Autodesk Inventor part; units mm, degrees
ref_plane "YZ Plane" through (0, 0, 0) normal (1, 0, 0) x (0, 1, 0)
ref_plane "XZ Plane" through (0, 0, 0) normal (0, 1, 0) x (-1, 0, 0)
ref_plane "XY Plane" through (0, 0, 0) normal (0, 0, 1) x (1, 0, 0)
sketch "Boceto1" plane through (0, 0, 0) normal (0, 0, 1) x (1, 0, 0)
  line L0 (0.9, -2.4) -> (-0.9, -2.4)
  line L1 (-0.9, -2.4) -> (-0.9, 2.4)
  line L2 (-0.9, 2.4) -> (0.9, 2.4)
  line L3 (0.9, 2.4) -> (0.9, -2.4)
  line L4 (0.9, -2.4) -> (-0.9, 2.4) construction
  line L5 (-0.9, -2.4) -> (0.9, 2.4) construction
  line L6 (2.4, -0.9) -> (-2.4, -0.9)
  line L7 (-2.4, -0.9) -> (-2.4, 0.9)
  line L8 (-2.4, 0.9) -> (2.4, 0.9)
  line L9 (2.4, 0.9) -> (2.4, -0.9)
  line L10 (2.4, -0.9) -> (-2.4, 0.9) construction
  line L11 (-2.4, -0.9) -> (2.4, 0.9) construction
  circle A0 centre (0, 0) radius 1.4
  point P0 (1.0724, 0.9)
  point P1 (0.9, 1.0724)
  point P2 (-0.9, 1.0724)
  point P3 (-1.0724, 0.9)
  point P4 (-1.0724, -0.9)
  point P5 (-0.9, -1.0724)
  point P6 (0.9, -1.0724)
  point P7 (1.0724, -0.9)
  dimension "d0" = 1.8
  dimension "d1" = 4.8
  dimension "d2" = 2.8
extrude "Extrusión1" add sketch "Boceto1" along normal blind 53
chamfer "Chaflán1" distance 0.2 angle 45 8 edges at (0.9, 2.4, 26.5) (2.4, 0.9, 26.5) (2.4, -0.9, 26.5) (0.9, -2.4, 26.5) (-0.9, 2.4, 26.5) (-2.4, 0.9, 26.5) (-2.4, -0.9, 26.5) (-0.9, -2.4, 26.5)
properties part number "EjeMotor"
For this review, take the finished solid that the model builds, in its own axes (mm). A direction names the side the tool comes from. Give positions to 0.01 mm unless a question says otherwise; leave off trailing zeros. Loops run counter-clockwise (first coordinate to the right, second up) from the corner with the lowest first, then second, coordinate; pieces in that order, holes last. Notation, with made-up numbers: M -18.5,18 L -11.5,18 A24 cw -11.5,40 Z; hole C 8,-20 d5. An arc over 180 degrees is marked long. Put each result on its own line as item: value. Start each with the question number.
(1) For pin 1 (0.6 mm diameter, centred on x = -2, z = 23.5, fed in from -Y); pin 2 (0.6 mm diameter, centred on y = 1.5, z = 22, fed in from +X); pin 3 (0.6 mm diameter, centred on y = -2, z = 30, fed in from -X), all flat-tipped, find the tip position at first contact; note any pin that passes through.
(2) Machinability: for faces 1 (the flat face through (-0.9, -2, 26)), 2 (the flat face through (-2, 0.9, 26)), 3 (the flat face through (0.9, -2, 26)), 4 (the flat face through (0, 2.4, 26)), 5 (the flat face through (0.9, 2, 26)), which of the approach directions +Z, -Z, +X, -X, +Y, -Y give a long, thin tool a straight path to every point of the face, cutting with its end or side? Answer none if there is none.
(3) Add section B-B, the plane y = 1.65. Write out the cut boundary in (x, z).
(4) Wall thickness on L1, parallel to X at y = -1.6, z = 37: over which ranges is the line inside the solid? List them lowest first.
(5) Add section A-A, the plane z = 22. Write out the cut boundary in (x, y), then the cut area to 3 significant figures.
Result:
1. pin 1: stops at y = -0.9
1. pin 2: stops at x = 0.9
1. pin 3: stops at x = -0.9
2. face 1: +Z, -Z, -X, -Y
2. face 2: +Z, -Z, -X, +Y
2. face 3: +Z, -Z, +X, -Y
2. face 4: +Z, -Z, +X, -X, +Y
2. face 5: +Z, -Z, +X, +Y
3. outline: M -0.9,0 L 0.9,0 L 0.9,53 L -0.9,53 Z
4. L1: x = -0.9 to 0.9
5. outline: M -2.4,-0.7 L -2.2,-0.9 L -1.07,-0.9 A1.4 ccw -0.9,-1.07 L -0.9,-2.2 L -0.7,-2.4 L 0.7,-2.4 L 0.9,-2.2 L 0.9,-1.07 A1.4 ccw 1.07,-0.9 L 2.2,-0.9 L 2.4,-0.7 L 2.4,0.7 L 2.2,0.9 L 1.07,0.9 A1.4 ccw 0.9,1.07 L 0.9,2.2 L 0.7,2.4 L -0.7,2.4 L -0.9,2.2 L -0.9,1.07 A1.4 ccw -1.07,0.9 L -2.2,0.9 L -2.4,0.7 Z
5. area: 13.9 mm^2
